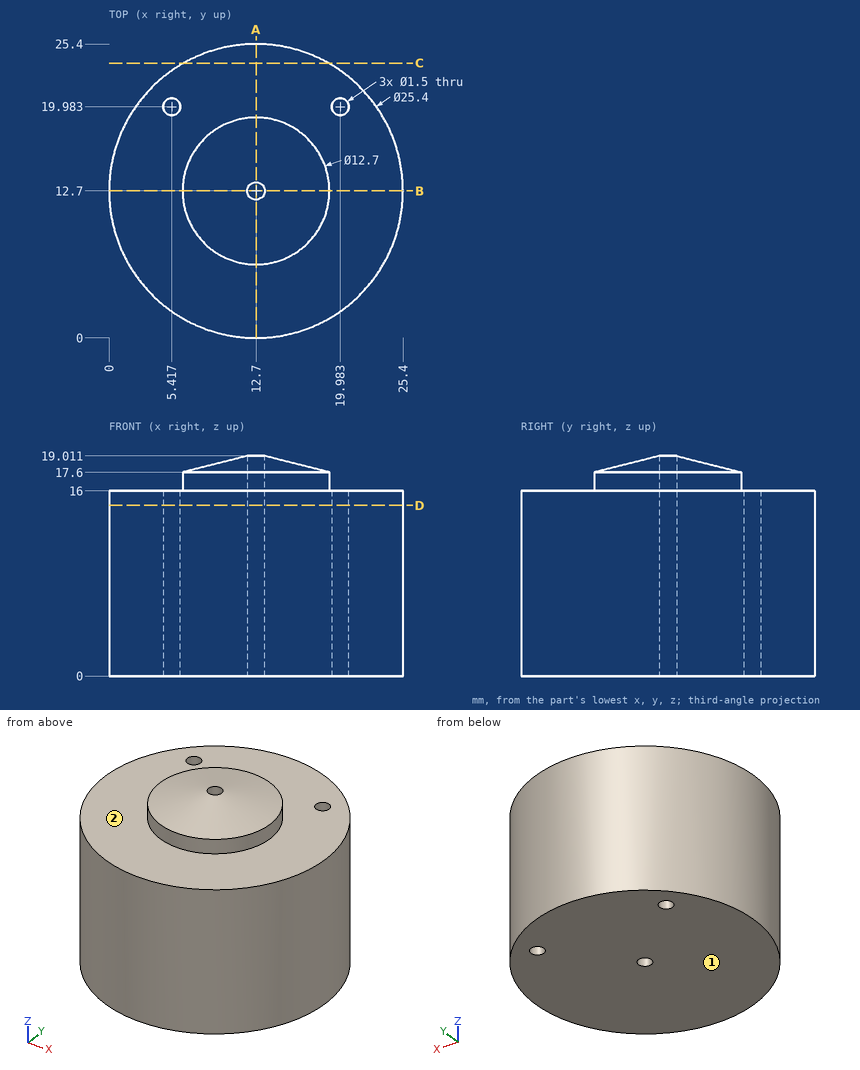
Print and shaded views of the part. All mm, measured from the part's lowest x, y and z. A direction names the side the tool comes from. Give positions to 0.01 mm unless a question says otherwise; leave off trailing zeros. Write each loop counter-clockwise with the first axis right and the second up, starting at its lowest first coordinate (ties: lowest second). Pieces come first, ordered by that corner, then holes. Notation, with made-up numbers: (-24.75, 58.5) - (-4.75, 58.5) arc R21 ccw to (-4.75, 88.5) - close; hole circle Ø7 at (-7, 11). An arc over 180 degrees is marked (long way). Put each result on its own line as item: value.
(1) Drop flat-ended pins along their axis: pin 1 Ø3 at (y, z) = (19.5, 8) entering from -X; pin 2 Ø4 at (y, z) = (7.5, 8.5) entering from -X; pin 3 Ø3 at (y, z) = (10, 15.5) entering from +X. Give the stop position or say it passes through.
Working result:
pin 1: x = 1.16
pin 2: x = 0.41
pin 3: x = 25.34
(2) Saw through at A-A (x = 12.7). List the corners of the cut face in (y, z), then the cut area to 3 significant figures.
Working result:
outline: (0, 0) - (11.95, 0) - (11.95, 19.01) - (6.35, 17.6) - (6.35, 16) - (0, 16) - close; (13.45, 0) - (25.4, 0) - (25.4, 16) - (19.05, 16) - (19.05, 17.6) - (13.45, 19.01) - close
area: 408 mm^2
(3) Saw through at C-C (y = 23.75). List the corners of the cut face in (x, z).
Working result:
outline: (6.44, 0) - (18.96, 0) - (18.96, 16) - (6.44, 16) - close
(4) Saw through at D-D (z = 14.75). List the corners of the cut face in (x, y), then the cut area to 3 significant figures.
Working result:
outline: circle Ø25.4 at (12.7, 12.7); hole circle Ø1.5 at (5.42, 19.98); hole circle Ø1.5 at (12.7, 12.7); hole circle Ø1.5 at (19.98, 19.98)
area: 501 mm^2
(5) Wall check: L1, parallel to Y at x = 12.7, z = 5.5; L2, parallel to Z at x = 14.25, y = 19.75; L3, parallel to Y at x = 7, z = 4.5. Give the ranges that are in metal, low to high.
Working result:
L1: 0 to 11.95, 13.45 to 25.4
L2: 0 to 16
L3: 1.35 to 24.05
(6) Tool access for the marked faces 1 and 2: list every direction of +Z, -Z, +X, -X, +Y, -Y with a clear straight run to the whole face (end or side of a thin tool).
Working result:
face 1: -Z, +X, -X, +Y, -Y
face 2: +Z
